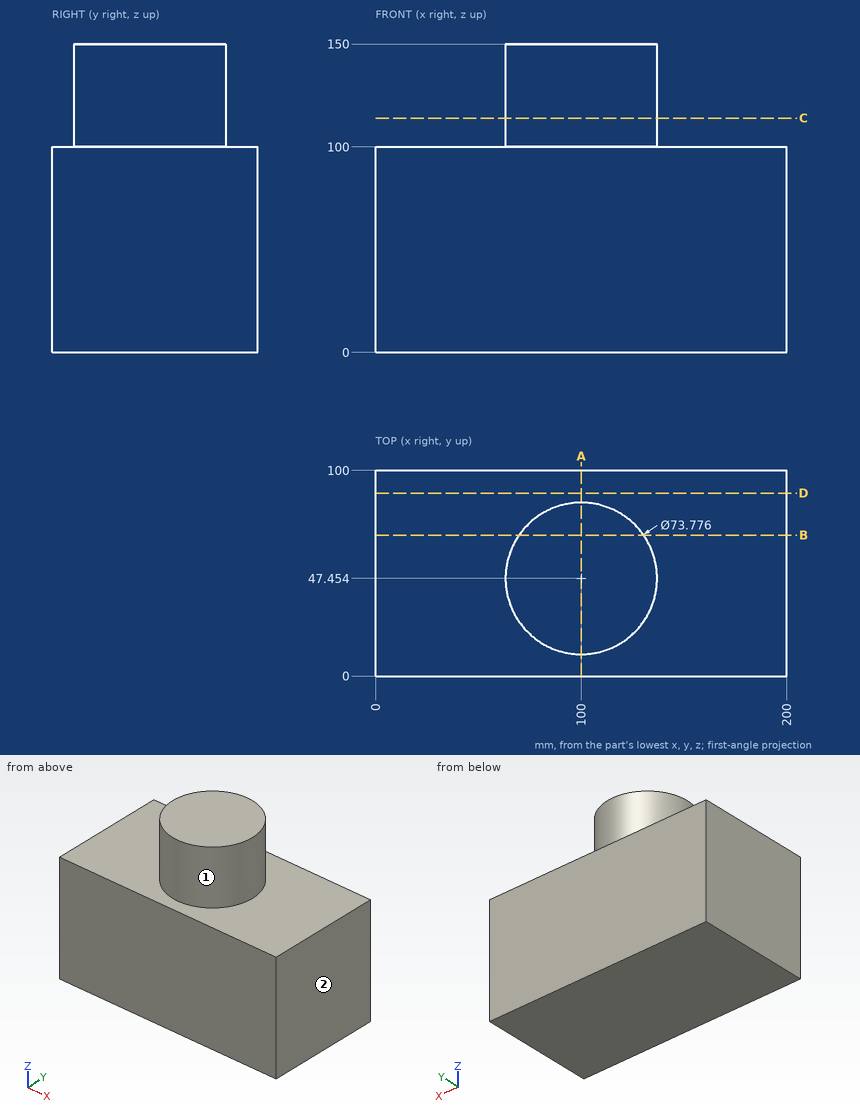
Design review of the part shown in the three views and the two pictorial views. Dimensions are in mm from the part's minimum x, y and z. A direction names the side the tool comes from. Round coordinates to 2 decimals unless told otherwise and drop trailing zeros. Order: outer loops, then holes, each group sorted by start corner. A loop starts at its lowest first (then second) coordinate and runs counter-clockwise, first axis right, second up.
Q1. We need section C-C, the plane z = 114. Give the boundary of the cut face in (x, y) (1 decimal), plus the area to 4 significant figures.
Findings below:
outline: circle Ø73.8 at (100, 47.5)
area: 4,275 mm2
Q2. Insertion check: P1, Ø4, axis at x = 163, y = 50, coming from the +Z side; P2, Ø8, axis at x = 116.5, z = 111, coming from the +Y side. Each pin has a flat end and moves straight along its axis. Give the tip position at first contact, or say it passes through.
Findings below:
P1: stops at z = 100
P2: stops at y = 82.16
Q3. Wall thickness on line 1 (Z direction, x = 184.5, y = 83); line 2 (X direction, y = 64.5, z = 140) (1 decimal); line 3 (X direction, y = 50, z = 107): over which ranges is each line inside the solid? List them lowest first.
Findings below:
line 1: z = 0 to 100
line 2: x = 67.3 to 132.7
line 3: x = 63.2 to 136.8
Q4. Machinability: for the marked faces 1 and 2, which of the approach directions +Z, -Z, +X, -X, +Y, -Y give a long, thin tool a straight path to every point of the face, cutting with its end or side? Answer none if there is none.
Findings below:
face 1: +Z
face 2: +Z, -Z, +X, +Y, -Y
Q5. We need section D-D, the plane y = 89. Give the boundary of the cut face in (x, z).
Findings below:
outline: (0, 0) - (200, 0) - (200, 100) - (0, 100) - close
Q6. We need section A-A, the plane x = 100. Give the boundary of the cut face in (y, z).
Findings below:
outline: (0, 0) - (100, 0) - (100, 100) - (84.34, 100) - (84.34, 150) - (10.57, 150) - (10.57, 100) - (0, 100) - close
Q7. We need section B-B, the plane y = 68.5. Give the boundary of the cut face in (x, z) (1 decimal), plus the area to 3 significant figures.
Findings below:
outline: (0, 0) - (200, 0) - (200, 100) - (130.3, 100) - (130.3, 150) - (69.7, 150) - (69.7, 100) - (0, 100) - close
area: 23,000 mm2
